Here's how the part is built. I have some questions about the finished solid (model axes, mm). A direction names the side the tool comes from. Coordinates: 2 decimals unless noted, no trailing zeros. Loops run counter-clockwise (first coordinate to the right, second up) from the corner with the lowest first, then second, coordinate; pieces in that order, holes last. Notation, with made-up numbers: M -28.75,6.25 L 16.25,6.25 A11 ccw 16.25,10.25 Z; hole C 21.5,47 d8. An arc over 180 degrees is marked long. Use one line per item in the form item = value. Start each with the question number.
(1) Thinking about a two-plate mould opening in X: for faces 4 (the flat face through (8, -4, 0)), 5 (the cylindrical face through (-6.367, 5.07, -0.303)), 6 (the flat face through (0, -7, 0)), 7 (the flat face through (-10, 4, 0)), which applies, +X half, -X half, draft (parallel to the pull), parting line (faces both ways), or undercut?
(2) Imagine slicing it at D-D, the plane z = 4. Please give me the cut outline in (x, y).
(3) Will these pins go through, and if not, where does the flat tip stop? P1, Ø5, axis at x = 5.5, z = 3.5, coming from the -Y side; P2, Ø0.7, axis at x = -5, z = -0.5, coming from the +Y side; P3, Ø6, axis at x = -2, y = -2.5, coming from the +Z side.
(4) Imagine slicing it at C-C, the plane z = -0.25. Please give me the cut outline in (x, y), and give its area (3 significant figures).
(5) Imagine slicing it at A-A, the plane x = 0. Please give me the cut outline in (y, z), and give its area (3 significant figures).
(6) Please list where these lines run through material, in increasing order: L1, parallel to X at y = 7.75, z = 0; L2, parallel to X at y = 1.5, z = 0; L3, parallel to Y at x = 0, z = 2.
(7) On a 3-axis mill with a long thin cutter (end or side, diameter ignored), from which of +Z, -Z, +X, -X, +Y, -Y can I reach the whole of each face in a straight line? I mean faces 1 (the cylindrical face through (6.39, 5.07, -0.18)), 2 (the flat face through (5.307, 3.007, 6.021)), 3 (the flat face through (10, 4, 0)). Say none if no direction works.
(8) Imagine slicing it at B-B, the plane y = 8.25. Please give me the cut outline in (x, z).
```python
from build123d import *

# Parameters (mm, degrees)
SKETCH_1_R          = 4.1
EXTRUDE_1_DEPTH     = 7.5
CUT_EXTRUDE_1_DEPTH = 3
SKETCH_3_R          = 1.4
CUT_EXTRUDE_4_DEPTH = 10


with BuildPart() as part:
    # 草图1 → 凸台-拉伸1 (new, symmetric)
    with BuildSketch(Plane.XY):
        Polygon((-10, 10), (10, 10), (10, -2), (5, -7), (-5, -7), (-10, -2), align=None)
        Circle(SKETCH_1_R, mode=Mode.SUBTRACT)
    extrude(amount=EXTRUDE_1_DEPTH, both=True)

    # 草图2 → 切除-拉伸1 (cut)
    with BuildSketch(Plane.XY.offset(7.5)):
        Polygon((7.043673284, 0), (3.521836642, 6.1), (-3.521836642, 6.1), (-7.043673284, 0), (-3.521836642, -6.1), (3.521836642, -6.1), align=None)
    extrude(amount=-CUT_EXTRUDE_1_DEPTH, mode=Mode.SUBTRACT)

    # 草图3 → 切除-拉伸4 (cut)
    with BuildSketch(Plane(origin=(0, 10, 0), x_dir=(1, 0, 0), z_dir=(0, 1, 0))):
        with Locations(Location((5, 0, 0), (0, 0, 270))):
            Circle(SKETCH_3_R)
        with Locations(Location((-5, 0, 0), (0, 0, 270))):
            Circle(SKETCH_3_R)
    extrude(amount=-CUT_EXTRUDE_4_DEPTH, mode=Mode.SUBTRACT)


solid = part.part
```
Answer:
q1.face_4 = +X half
q1.face_5 = undercut
q1.face_6 = draft
q1.face_7 = -X half
q2.outline = M -10,-2 L -5,-7 L 5,-7 L 10,-2 L 10,10 L -10,10 Z; hole C 0,0 d8.2
q3.P1 = -7
q3.P2 = 0
q3.P3 = 4.5
q4.outline = M -10,-2 L -5,-7 L 5,-7 L 10,-2 L 10,10 L 6.38,10 L 6.38,0 L 4.1,0 A4.1 cw -4.1,0 L -6.38,0 L -6.38,10 L -10,10 Z; M -3.62,1.92 A4.1 cw 3.62,1.92 L 3.62,10 L -3.62,10 Z
q4.area = 208 mm²
q5.outline = M -7,-7.5 L -4.1,-7.5 L -4.1,4.5 L -6.1,4.5 L -6.1,7.5 L -7,7.5 Z; M 4.1,-7.5 L 10,-7.5 L 10,7.5 L 6.1,7.5 L 6.1,4.5 L 4.1,4.5 Z
q5.area = 120 mm²
q6.L1 = -10 to -6.4, -3.6 to 3.6, 6.4 to 10
q6.L2 = -10 to -6.4, 6.4 to 10
q6.L3 = -7 to -4.1, 4.1 to 10
q7.face_1 = +Y
q7.face_2 = +Z
q7.face_3 = +Z, -Z, +X, +Y, -Y
q8.outline = M -10,-7.5 L 10,-7.5 L 10,7.5 L -10,7.5 Z; hole C -5,0 d2.8; hole C 5,0 d2.8
